Geometry: final body of the model. Coordinates: model frame, mm. Face numbers are marked on the shaded views. A direction names the side the tool comes from. Coordinates: 2 decimals unless noted, no trailing zeros. Order: outer loops, then holes, each group sorted by start corner. A loop starts at its lowest first (then second) coordinate and runs counter-clockwise, first axis right, second up. Notation, with made-up numbers: (69.5, 71.25) - (122.5, 71.25) arc R15 ccw to (122.5, 93.25) - close; hole circle Ø7 at (55.5, -4). An arc over 180 degrees is marked (long way). Use one line per item in the form item = value. Start each with the question number.
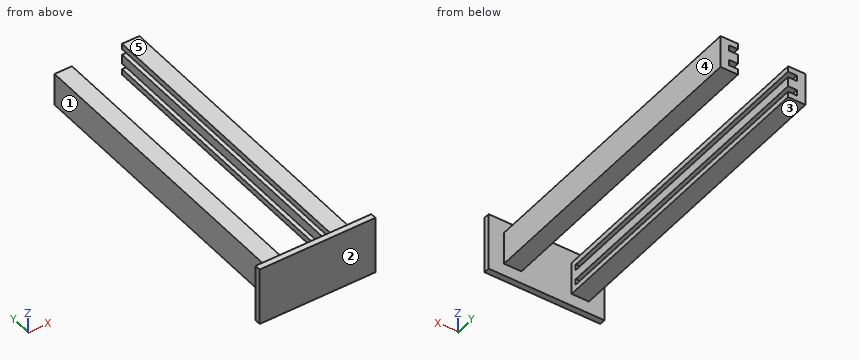
```python
from build123d import *

# Parameters (mm, degrees)
SKETCH1_W           = 60
SKETCH1_H           = 30
BOSS_EXTRUDE1_DEPTH = 3
SKETCH2_W           = 9
SKETCH2_H           = 17
BOSS_EXTRUDE2_DEPTH = 160
SKETCH3_W           = 4.5
SKETCH3_H           = 3
CUT_EXTRUDE1_DEPTH  = 157


with BuildPart() as part:
    # Sketch1 → Boss-Extrude1 (new body)
    with BuildSketch(Plane(origin=(0, 0, 0), x_dir=(1, 0, 0), z_dir=(0, 1, 0))):
        Rectangle(SKETCH1_W, SKETCH1_H)
    extrude(amount=BOSS_EXTRUDE1_DEPTH)

    # Sketch2 → Boss-Extrude2 (add)
    with BuildSketch(Plane(origin=(0, 3, 0), x_dir=(1, 0, 0), z_dir=(0, 1, 0))):
        with Locations((17.5, 0)):
            Rectangle(SKETCH2_W, SKETCH2_H)
        with Locations((-17.5, 0)):
            Rectangle(SKETCH2_W, SKETCH2_H)
    extrude(amount=BOSS_EXTRUDE2_DEPTH)

    # Sketch3 → Cut-Extrude1 (cut)
    with BuildSketch(Plane(origin=(0, 163, 0), x_dir=(1, 0, 0), z_dir=(0, 1, 0))):
        with Locations((-15.25, 4)):
            Rectangle(SKETCH3_W, SKETCH3_H)
        with Locations((-15.25, -4)):
            Rectangle(SKETCH3_W, SKETCH3_H)
        with Locations((15.25, -4)):
            Rectangle(SKETCH3_W, SKETCH3_H)
        with Locations((15.25, 4)):
            Rectangle(SKETCH3_W, SKETCH3_H)
    extrude(amount=-CUT_EXTRUDE1_DEPTH, mode=Mode.SUBTRACT)


solid = part.part
```
(1) Cut plane C-C on z = 0.25. Return the cut outline in (x, y), plus the area to 3 significant figures.
(2) Contact query for flat-ended pins moving along their axis: pin 1 Ø13.5 at (y, z) = (53.5, 3) entering from +X; pin 2 Ø3 at (y, z) = (20, -7.5) entering from -X; pin 3 Ø5 at (x, y) = (-16, 113.5) entering from -Z. Output: stop coordinate, or through.
(3) Cut plane D-D on z = -10. Return the cut outline in (x, y), plus the area to 3 significant figures.
(4) Cut plane B-B on x = 19. Return the cut outline in (y, z), plus the area to 3 significant figures.
(5) Set-up query: the marked faces 1, 2, 3, 4 and 5. Return all of +Z, -Z, +X, -X, +Y, -Y with unobstructed straight access to the full face (end or side cutting, diameter ignored); none if empty.
(6) Cut plane A-A on y = 66. Return the cut outline in (x, z).
(7) Material intervals for L1, parallel to Z at x = -17, y = 120; L2, parallel to X at y = 148.5, z = -4.5; L3, parallel to X at y = 154.5, z = 1.25, sorted ascending. Write a range as from..to.
Check sheet entries:
q1.outline = (-30, 0) - (30, 0) - (30, 3) - (22, 3) - (22, 163) - (13, 163) - (13, 3) - (-13, 3) - (-13, 163) - (-22, 163) - (-22, 3) - (-30, 3) - close
q1.area = 3,060 mm^2
q2.pin_1 = 22
q2.pin_2 = -22
q2.pin_3 = -8.5
q3.outline = (-30, 0) - (30, 0) - (30, 3) - (-30, 3) - close
q3.area = 180 mm^2
q4.outline = (0, -15) - (3, -15) - (3, -8.5) - (163, -8.5) - (163, 8.5) - (3, 8.5) - (3, 15) - (0, 15) - close
q4.area = 2,810 mm^2
q5.face_1 = +Z, -Z, -X, +Y
q5.face_2 = +Z, -Z, +X, -X, -Y
q5.face_3 = -Z, +X, -X, +Y
q5.face_4 = +Z, -Z, +X, +Y
q5.face_5 = +Z, +X, -X, +Y
q6.outline = (-22, -8.5) - (-13, -8.5) - (-13, -5.5) - (-17.5, -5.5) - (-17.5, -2.5) - (-13, -2.5) - (-13, 2.5) - (-17.5, 2.5) - (-17.5, 5.5) - (-13, 5.5) - (-13, 8.5) - (-22, 8.5) - close; (13, -8.5) - (22, -8.5) - (22, 8.5) - (13, 8.5) - (13, 5.5) - (17.5, 5.5) - (17.5, 2.5) - (13, 2.5) - (13, -2.5) - (17.5, -2.5) - (17.5, -5.5) - (13, -5.5) - close
q7.L1 = -8.5..-5.5, -2.5..2.5, 5.5..8.5
q7.L2 = -22..-17.5, 17.5..22
q7.L3 = -22..-13, 13..22
